For this review, take the finished solid that the model builds, in its own axes (mm). Round coordinates to 2 decimals unless told otherwise and drop trailing zeros. Loops run counter-clockwise (first coordinate to the right, second up) from the corner with the lowest first, then second, coordinate; pieces in that order, holes last.
1) Take a section at B-B (y = -6). State the section outline as (x, z) points, then the cut area to 3 significant figures.
2) Take a section at A-A (y = -29). State the section outline as (x, z) points, then the cut area to 3 significant figures.
3) Take a section at C-C (x = -1). State the section outline as (y, z) points.
4) Insertion check: pin 1 (0.8 mm diameter, centred on x = 31.5, z = 1, fed in from +Y); pin 2 (0.5 mm diameter, centred on x = 30, z = 1, fed in from -Y); pin 3 (8 mm diameter, centred on x = -5.5, y = 27.5, fed in from +Z). Each pin has a flat end and moves straight along its axis. Give the tip position at first contact, or say it passes through.
5) Take a section at D-D (y = 32). State the section outline as (x, z) points, then the cut area to 3 significant figures.
6) Wall thickness on L1, parallel to X at y = -6, z = 0.75; L2, parallel to X at y = 16.5, z = 1.2; L3, parallel to X at y = -20, z = 0.1: over which ranges is each line inside the solid? List them lowest first.
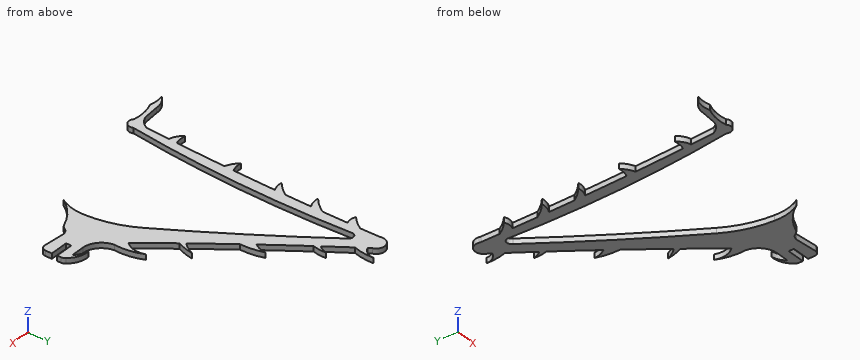
```python
from build123d import *

# Parameters (mm, degrees)
BOSS_EXTRUDE1_DEPTH = 1.524


with BuildPart() as part:
    # Sketch1 → Boss-Extrude1 (new body)
    with BuildSketch(Plane.XY):
        with BuildLine():
            Line((-24.364554891, -37.477178577), (-29.107446573, -37.903411516))
            ThreePointArc((-29.107446573, -37.903411516), (-31.473071099, -38.393425652), (-33.42606857, -39.815429216))
            ThreePointArc((-33.42606857, -39.815429216), (-31.249893388, -39.522353453), (-29.073637755, -39.814831212))
            ThreePointArc((-29.073637755, -39.814831212), (-25.648712592, -38.918813581), (-22.109711099, -39.010619897))
            ThreePointArc((-22.109711099, -39.010619897), (-19.760509062, -39.158760526), (-19.17540942, -36.878770555))
            ThreePointArc((-19.17540942, -36.878770555), (-15.865162798, -3.599783912), (-15.772880419, 29.843304591))
            ThreePointArc((-15.772880419, 29.843304591), (-14.548235849, 30.854621423), (-13.192137962, 30.027872017))
            ThreePointArc((-13.192137962, 30.027872017), (-0.136306851, 10.515149008), (12.117439823, -9.511003335))
            ThreePointArc((12.117439823, -9.511003335), (14.987237528, -16.164940717), (16.168465676, -23.314438715))
            ThreePointArc((16.168465676, -23.314438715), (15.842573186, -27.376128515), (14.280506414, -31.139568078))
            ThreePointArc((14.280506414, -31.139568078), (17.769072475, -27.290062934), (22.267530319, -24.691474848))
            ThreePointArc((22.267530319, -24.691474848), (23.021800675, -24.236514222), (23.57532619, -23.551297143))
            ThreePointArc((23.57532619, -23.551297143), (24.39123878, -22.713681417), (25.519929239, -22.408114227))
            Line((25.519929239, -22.408114227), (31.91215665, -22.925682288))
            ThreePointArc((31.91215665, -22.925682288), (32.987506925, -22.470894628), (33.426022068, -21.3888066))
            Line((33.426022068, -21.3888066), (33.414100594, -19.560808287))
            Line((33.414100594, -19.560808287), (28.122840134, -19.561801701))
            Line((28.122840134, -19.561801701), (28.110918151, -18.035820501))
            Line((28.110918151, -18.035820501), (33.406152775, -18.035820501))
            Line((33.406152775, -18.035820501), (33.398174437, -16.925455032))
            ThreePointArc((33.398174437, -16.925455032), (33.278622124, -16.341687991), (32.944745486, -15.848126338))
            ThreePointArc((32.944745486, -15.848126338), (30.558622948, -13.902263693), (27.514270045, -13.441962054))
            ThreePointArc((27.514270045, -13.441962054), (29.473047609, -14.099689708), (31.069176316, -15.411859044))
            Line((31.069176316, -15.411859044), (27.131733148, -15.435585668))
            ThreePointArc((27.131733148, -15.435585668), (23.499650774, -13.970182339), (21.752807973, -10.464762321))
            ThreePointArc((21.752807973, -10.464762321), (21.619864509, -6.287804949), (20.411069114, -2.287372404))
            ThreePointArc((20.411069114, -2.287372404), (20.646164492, -5.489635666), (19.164832874, -8.338392672))
            ThreePointArc((19.164832874, -8.338392672), (15.589025091, -3.695796166), (12.046655257, 0.972364027))
            ThreePointArc((12.046655257, 0.972364027), (12.956062916, 3.299009299), (13.502748407, 5.736515296))
            ThreePointArc((13.502748407, 5.736515296), (12.481630447, 3.853470902), (11.130205062, 2.191487897))
            ThreePointArc((11.130205062, 2.191487897), (7.442893614, 7.145097778), (3.793181539, 12.12647493))
            ThreePointArc((3.793181539, 12.12647493), (3.6391771, 15.54128121), (2.898904085, 18.878437958))
            ThreePointArc((2.898904085, 18.878437958), (2.513226677, 16.946929667), (1.548714149, 15.229609975))
            ThreePointArc((1.548714149, 15.229609975), (-2.262432259, 20.570077326), (-6.030509674, 25.941019614))
            ThreePointArc((-6.030509674, 25.941019614), (-5.660787122, 27.892481118), (-5.62524637, 29.878339526))
            ThreePointArc((-5.62524637, 29.878339526), (-6.161870131, 28.501450031), (-6.932604962, 27.240594145))
            ThreePointArc((-6.932604962, 27.240594145), (-9.183193775, 30.506482698), (-11.417879239, 33.783273646))
            ThreePointArc((-11.417879239, 33.783273646), (-10.755972391, 36.763721595), (-10.665026003, 39.815429216))
            ThreePointArc((-10.665026003, 39.815429216), (-11.282248363, 37.628788529), (-13.063123372, 36.21781541))
            ThreePointArc((-13.063123372, 36.21781541), (-13.355981093, 36.653158865), (-13.648558784, 37.088690566))
            ThreePointArc((-13.648558784, 37.088690566), (-16.663200217, 38.770611805), (-18.464850886, 35.825959552))
            ThreePointArc((-18.464850886, 35.825959552), (-18.420691896, 35.556546257), (-18.405703646, 35.283949682))
            ThreePointArc((-18.405703646, 35.283949682), (-18.40664027, 32.572114189), (-18.415743017, 29.860293811))
            ThreePointArc((-18.415743017, 29.860293811), (-19.802823987, 27.891016102), (-21.515118511, 26.1968804))
            ThreePointArc((-21.515118511, 26.1968804), (-19.981611623, 25.800865516), (-18.441254033, 26.16933486))
            ThreePointArc((-18.441254033, 26.16933486), (-18.482213638, 22.453964053), (-18.538502103, 18.738793864))
            ThreePointArc((-18.538502103, 18.738793864), (-20.176761137, 16.529345851), (-22.151609818, 14.614789539))
            ThreePointArc((-22.151609818, 14.614789539), (-20.30809135, 14.67247237), (-18.602694106, 15.374973539))
            ThreePointArc((-18.602694106, 15.374973539), (-18.691127928, 11.543467884), (-18.795866803, 7.712373276))
            ThreePointArc((-18.795866803, 7.712373276), (-20.334999659, 5.725783654), (-22.151609818, 3.989294148))
            ThreePointArc((-22.151609818, 3.989294148), (-20.47435397, 4.014209715), (-18.893763009, 4.575939347))
            ThreePointArc((-18.893763009, 4.575939347), (-19.121395234, -1.672175675), (-19.392400358, -7.918559748))
            ThreePointArc((-19.392400358, -7.918559748), (-21.046264617, -8.374679978), (-22.761865121, -8.369430126))
            ThreePointArc((-22.761865121, -8.369430126), (-21.306272714, -9.735931232), (-19.523833936, -10.635368018))
            ThreePointArc((-19.523833936, -10.635368018), (-19.916786026, -17.918683373), (-20.36871487, -25.198577206))
            ThreePointArc((-20.36871487, -25.198577206), (-22.05068144, -25.516497621), (-23.761121477, -25.44956621))
            ThreePointArc((-23.761121477, -25.44956621), (-22.378228066, -26.891420245), (-20.535063915, -27.662188146))
            ThreePointArc((-20.535063915, -27.662188146), (-20.777686634, -31.088285528), (-21.033374555, -34.513432641))
            ThreePointArc((-21.033374555, -34.513432641), (-22.397678986, -36.333943653), (-24.364554891, -37.477178577))
        make_face()
    extrude(amount=BOSS_EXTRUDE1_DEPTH)


solid = part.part
```
Response:
1. outline: (-19.3, 0) - (-16, 0) - (-16, 1.52) - (-19.3, 1.52) - close; (10.05, 0) - (17.36, 0) - (17.36, 1.52) - (10.05, 1.52) - close; (20.52, 0) - (21.57, 0) - (21.57, 1.52) - (20.52, 1.52) - close
1. area: 17.8 mm2
2. outline: (-20.63, 0) - (-18.1, 0) - (-18.1, 1.52) - (-20.63, 1.52) - close; (15.34, 0) - (15.95, 0) - (15.95, 1.52) - (15.34, 1.52) - close
2. area: 4.79 mm2
3. outline: (11.86, 0) - (18.79, 0) - (18.79, 1.52) - (11.86, 1.52) - close
4. pin 1: stops at y = -14.18
4. pin 2: stops at y = -22.79
4. pin 3: stops at z = 1.52
5. outline: (-18.41, 0) - (-10.2, 0) - (-10.2, 1.52) - (-18.41, 1.52) - close
5. area: 12.5 mm2
6. L1: x = -19.3 to -16, 10.05 to 17.36, 20.52 to 21.57
6. L2: x = -20.2 to -15.42, -4.02 to 0.64, 2.33 to 3.49
6. L3: x = -20.04 to -17.09, 15.84 to 33.42
